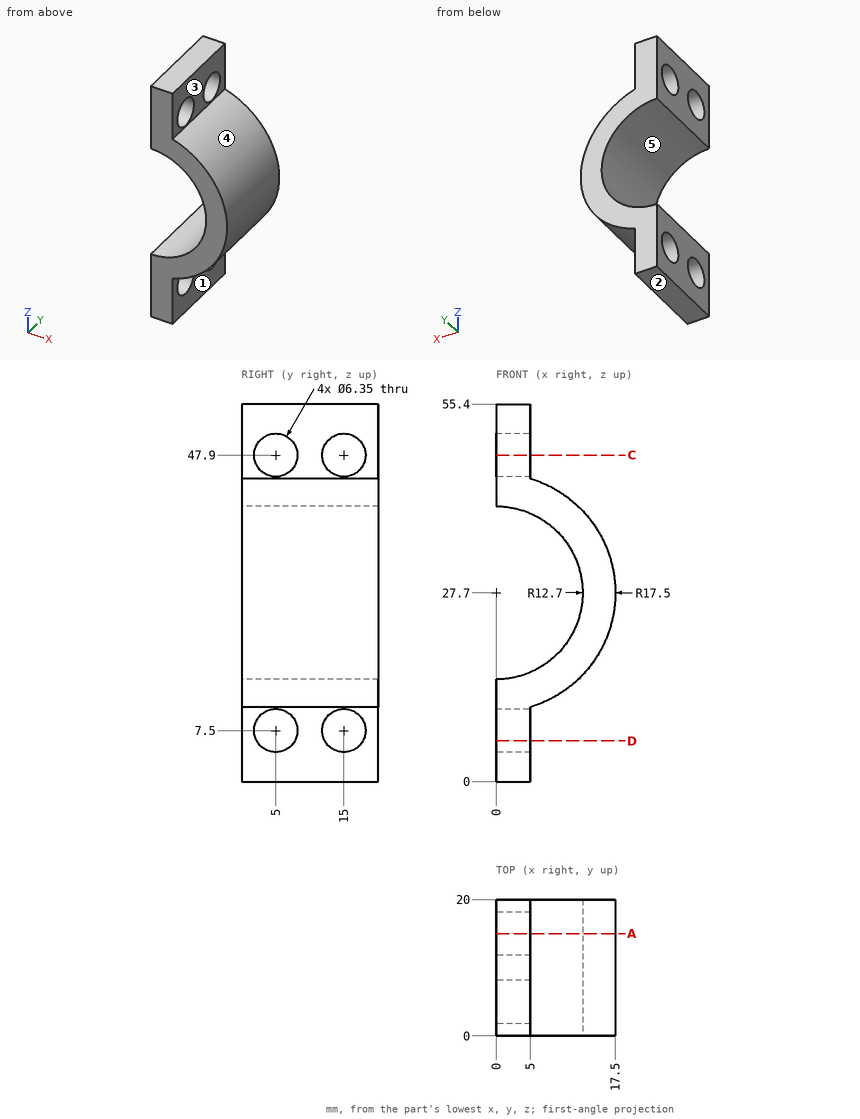
Print and shaded views of the part. All mm, measured from the part's lowest x, y and z. A direction names the side the tool comes from. Give positions to 0.01 mm unless a question says otherwise; leave off trailing zeros. Write each loop counter-clockwise with the first axis right and the second up, starting at its lowest first coordinate (ties: lowest second). Pieces come first, ordered by that corner, then holes. Notation, with made-up numbers: (42, 65) -> (67, 65) arc R15 cw to (67, 82) -> close; hole circle Ø9 at (28, 31.25). An arc over 180 degrees is marked (long way). Write each question's results on one line, items separated by ' | '.
1. Wall check: probe 1 along Y at (x, z) = (1.6, 47.9) (3 decimals); probe 2 along Z at (x, y) = (1.75, 12.5); probe 3 along Z at (x, y) = (8, 1.5). Give the ranges that are in metal, low to high. Write a range as [from, to].
Geometry check:
probe 1: [0, 1.825], [8.175, 11.825], [18.175, 20] | probe 2: [0, 5.54], [9.46, 15.12], [40.28, 45.94], [49.86, 55.4] | probe 3: [12.14, 17.84], [37.56, 43.26]
2. Drop flat-ended pins along their axis: P1, Ø3, axis at x = 4, y = 11.5, coming from the -Z side; P2, Ø3.5, axis at y = 12.5, z = 48.5, coming from the +X side; P3, Ø4, axis at y = 3.5, z = 20.5, coming from the -X side (3 decimals); P4, Ø10, axis at y = 5, z = 7.5, coming from the +X side. Give the stop position or say it passes through.
Geometry check:
P1: z = 0 | P2: x = 5 | P3: x = 8.755 | P4: x = 8.67
3. Two-plate mould, pull along Z, no slides. Class the marked faces 3, 4 and 5: pulls with the +Z half, pulls with the -Z half, needs draft (parallel to the pull), parting line crosses it, or undercut.
Geometry check:
face 3: needs draft | face 4: parting line crosses it | face 5: undercut
4. Cut at C-C, the plane z = 47.9. Write the cut outline in (x, y) (3 decimals), then the cut area to 3 significant figures.
Geometry check:
outline: (0, 0) -> (5, 0) -> (5, 1.825) -> (0, 1.825) -> close; (0, 8.175) -> (5, 8.175) -> (5, 11.825) -> (0, 11.825) -> close; (0, 18.175) -> (5, 18.175) -> (5, 20) -> (0, 20) -> close | area: 36.5 mm²
5. Cut at A-A, the plane y = 15. Give the number of separate pieces and of enclosed holes in the cut face, then the cut area to 3 significant figures.
Geometry check:
separate pieces: 3 | enclosed holes: 0 | area: 269 mm²
6. Which spindle directions (+Z, -Z, +X, -X, +Y, -Y) get a long thin tool onto all of the face, cutting with end or side? Do the marked faces 1 and 2. Say none if no direction does.
Geometry check:
face 1: -Z, +X, +Y, -Y | face 2: -Z, +X, -X, +Y, -Y
7. Cut at D-D, the plane z = 6. Write the cut outline in (x, y), then the cut area to 3 significant figures.
Geometry check:
outline: (0, 0) -> (5, 0) -> (5, 2.2) -> (0, 2.2) -> close; (0, 7.8) -> (5, 7.8) -> (5, 12.2) -> (0, 12.2) -> close; (0, 17.8) -> (5, 17.8) -> (5, 20) -> (0, 20) -> close | area: 44.0 mm²
